Geometry check sheet. Reference: the model listing, model coordinates, mm. A direction names the side the tool comes from. Give positions to 0.01 mm unless a question says otherwise; leave off trailing zeros. Loops run counter-clockwise (first coordinate to the right, second up) from the corner with the lowest first, then second, coordinate; pieces in that order, holes last. Notation, with made-up numbers: (-32, 27.25) -> (10, 27.25) arc R19 ccw to (10, 61.25) -> close; hole circle Ø5 at (-6.75, 57.5). An arc over 180 degrees is marked (long way). Write item = value, one per line.
```python
from build123d import *

# Parameters (mm, degrees)
SKETCH1_R           = 30
BOSS_EXTRUDE1_DEPTH = 25
BOSS_EXTRUDE2_DEPTH = 50
SKETCH4_W           = 10
SKETCH4_H           = 10
BOSS_EXTRUDE3_DEPTH = 30


with BuildPart() as part:
    # Sketch1 → Boss-Extrude1 (new body)
    with BuildSketch(Plane(origin=(0, 0, 0), x_dir=(1, 0, 0), z_dir=(0, 1, 0))):
        Circle(SKETCH1_R)
    extrude(amount=BOSS_EXTRUDE1_DEPTH)

    # Sketch3 → Boss-Extrude2 (add)
    with BuildSketch(Plane(origin=(0, 25, 0), x_dir=(1, 0, 0), z_dir=(0, 1, 0))):
        Polygon((-15, 0.769018566), (-15, 15), (15, 15), (15, -15), (-15, -15), align=None)
    extrude(amount=BOSS_EXTRUDE2_DEPTH)

    # Sketch4 → Boss-Extrude3 (add)
    with BuildSketch(Plane(origin=(0, 75, 0), x_dir=(1, 0, 0), z_dir=(0, 1, 0))):
        Rectangle(SKETCH4_W, SKETCH4_H)
    extrude(amount=BOSS_EXTRUDE3_DEPTH)

    # Sketch7 → Revolve1 (revolve)
    with BuildSketch(Plane(origin=(0, 110, 0), x_dir=(1, 0, 0), z_dir=(0, 1, 0))):
        with BuildLine():
            Line((0, 11.606043258), (0, -11.606043258))
            ThreePointArc((0, -11.606043258), (11.606043258, 0), (0, 11.606043258))
        make_face()
    revolve(axis=Axis((0, 110, -11.606043258), (0, 0, 1)))


solid = part.part
```
Item 1: Section check A-A, the plane z = 9.5. Record the cut outline in (x, y).
Answer:
outline = (-28.46, 0) -> (28.46, 0) -> (28.46, 25) -> (15, 25) -> (15, 75) -> (-15, 75) -> (-15, 25) -> (-28.46, 25) -> close; circle Ø13.33 at (0, 110)
Item 2: Section check C-C, the plane y = 82.5. Record the cut outline in (x, z).
Answer:
outline = (-5, -5) -> (5, -5) -> (5, 5) -> (-5, 5) -> close
Item 3: Section check B-B, the plane x = -9. Record the cut outline in (y, z).
Answer:
outline = (0, -28.62) -> (25, -28.62) -> (25, -15) -> (75, -15) -> (75, 15) -> (25, 15) -> (25, 28.62) -> (0, 28.62) -> close; circle Ø14.66 at (110, 0)
Item 4: Section check D-D, the plane z = 0. Record the cut outline in (x, y), plus the area to 3 significant figures.
Answer:
outline = (-30, 0) -> (30, 0) -> (30, 25) -> (15, 25) -> (15, 75) -> (5, 75) -> (5, 99.53) arc R11.61 ccw (long way) to (-5, 99.53) -> (-5, 75) -> (-15, 75) -> (-15, 25) -> (-30, 25) -> close
area = 3,660 mm^2
Item 5: Thickness scan on L1, parallel to X at y = 41, z = -6; L2, parallel to Z at x = 3.5, y = 86. Record the ranges inside material, lowest first. Write a range as [from, to].
Answer:
L1 = [-15, 15]
L2 = [-5, 5]
Item 6: Draft check along Y on faces 4 (the flat face through (0, 50, -15)), 5 (the flat face through (0, 0, 0)), 6 (the flat face through (5, 88, 0)). Enter one of: +Y half, -Y half, draft (parallel to the pull), parting line (faces both ways), or undercut.
Answer:
face_4 = draft
face_5 = -Y half
face_6 = undercut
Item 7: Gauge pin test, flat ends, axial feed: pin 1 (18 mm diameter, centred on x = -12.5, z = -11.5, fed in from +Y); pin 2 (4 mm diameter, centred on x = -19.5, z = 10.5, fed in from +Y); pin 3 (8 mm diameter, centred on x = -0.5, y = 87, fed in from +Z). Record the tip position at first contact, or that the pin passes through.
Answer:
pin_1 = 118.42
pin_2 = 25
pin_3 = 5
Item 8: Tool access check on faces 1 (the flat face through (7, 75, 0)), 2 (the flat face through (0, 50, 15)), 3 (the flat face through (15, 50, 0)). Record the directions out of +Z, -Z, +X, -X, +Y, -Y that give a thin tool (end or side, any length) a straight path to the whole face; none if there is none.
Answer:
face_1 = none
face_2 = +Z, +X, -X, +Y
face_3 = +Z, -Z, +X, +Y
